```python
from build123d import *

# Parameters (mm, degrees)
F0_R           = 15
F1_DEPTH       = 3.6
F2_R           = 12
F3_DEPTH       = 10.5
F5_D           = 6.8
F5_CSINK_D     = 17.92
F5_CSINK_ANGLE = 90
F6_W           = 3.6
F6_H           = 5
F8_SIZE        = 0.25
F9_R           = 2
F10_SIZE       = 2
F11_R          = 5
F12_DEPTH      = 8


with BuildPart() as f1:
    # F0 (on Right) → F1 (new body)
    with BuildSketch(Plane.YZ):
        Circle(F0_R)
    extrude(amount=F1_DEPTH)

    # F2 (on face) → F3 (join)
    with BuildSketch(Plane.YZ.offset(3.6)):
        Circle(F2_R)
    extrude(amount=F3_DEPTH)

    # F5 (through all)
    with Locations(Plane.YZ.offset(14.1)):
        with Locations((0, 0)):
            CounterSinkHole(F5_D / 2, F5_CSINK_D / 2, counter_sink_angle=F5_CSINK_ANGLE)

    # F6 (on Front) → F7 (revolve, cut)
    with BuildSketch(Plane.XZ):
        with Locations((5.4, 10.5)):
            Rectangle(F6_W, F6_H)
    revolve(axis=Axis((8.5571676374, 0, 0), (1, 0, 0)), mode=Mode.SUBTRACT)

    # F8
    f8_edges = [f1.edges().sort_by_distance(p)[0] for p in [
        (0, -15, 0),
        (7.2, -12, 0),
    ]]
    chamfer(f8_edges, length=F8_SIZE)

    # F9
    f9_edges = [f1.edges().sort_by_distance(p)[0] for p in [
        (3.6, -15, 0),
    ]]
    fillet(f9_edges, radius=F9_R)

    # F10
    f10_edges = [f1.edges().sort_by_distance(p)[0] for p in [
        (14.1, -12, 0),
    ]]
    chamfer(f10_edges, length=F10_SIZE)

    # F11 (on face) → F12 (cut)
    with BuildSketch(Plane.YZ.offset(14.1)):
        Circle(F11_R)
    extrude(amount=-F12_DEPTH, mode=Mode.SUBTRACT)


solid = f1.part
```
Here's how the part is built. I have some questions about the finished solid (model axes, mm). A direction names the side the tool comes from. Coordinates: 2 decimals unless noted, no trailing zeros. Write each loop counter-clockwise with the first axis right and the second up, starting at its lowest first coordinate (ties: lowest second). Pieces come first, ordered by that corner, then holes. Notation, with made-up numbers: (44, -34) -> (76, -34) arc R11 ccw to (76, -19) -> close; hole circle Ø10 at (-36.75, 51.25). An arc over 180 degrees is marked (long way). Use a Markdown table: item, result. Add a question column.
(1) If we section it at D-D, the plane x = 2: Write out the boundary of the cut face in (y, z).
(2) We'd pull the mould along Y, two halves only. Please class faces 1 (the cylindrical face through (5.43, 7.81, -1.73)), 2 (the cylindrical face through (8.15, -1.08, -4.88)), 3 (the flat face through (7.2, 8, -2)), 4 (the conical face through (10.332, 1.126, -5.069)): +Y half, -Y half, draft (parallel to the pull), parting line (faces both ways), or undercut.
(3) Please list where these lines run through material, in increasing order: line 1 (Z direction, x = 1.75, y = 0); line 2 (Z direction, x = 4.25, y = 0); line 3 (Y direction, x = 7, z = 0).
(4) For faces 5 (the flat face through (3.6, 6, 6)), 6 (the cylindrical face through (3.01, 0.74, -3.32)), 7 (the cylindrical face through (9.74, -11.99, 0.53)), which set-ups out of +Z, -Z, +X, -X, +Y, -Y let a thin tool reach every point of the face, with its end or its side?
(5) I'm going to push flat-ended pins straight in: P1, Ø1.5, axis at x = 3.5, z = 1.5, coming from the +Y side; P2, Ø4, axis at x = 6, y = -3, coming from the -Z side; P3, Ø8, axis at y = 0, z = 0, coming from the +X side; P4, Ø10, axis at y = 8.5, z = 1, coming from the +X side. Where does each tip first touch, or does it pass through?
(6) If we section it at C-C, the plane x = 10.5: Write out the boundary of the cut face in (y, z).
Outcome:
| question | item | result |
|---|---|---|
| 1 | outline | circle Ø29.92 at (0, 0); hole circle Ø6.8 at (0, 0) |
| 2 | face 1 | parting line |
| 2 | face 2 | undercut |
| 2 | face 3 | draft |
| 2 | face 4 | undercut |
| 3 | line 1 | z = -14.99 to -3.4, 3.4 to 14.99 |
| 3 | line 2 | z = -8 to -3.4, 3.4 to 8 |
| 3 | line 3 | y = -8 to -5, 5 to 8 |
| 4 | face 5 | none |
| 4 | face 6 | +X, -X |
| 4 | face 7 | +X |
| 5 | P1 | stops at y = 14.56 |
| 5 | P2 | stops at z = -11.89 |
| 5 | P3 | stops at x = 6.1 |
| 5 | P4 | stops at x = 14.1 |
| 6 | outline | circle Ø24 at (0, 0); hole circle Ø10.72 at (0, 0) |
